CAD build for the part. Positions are in the model's coordinates, mm. Give positions to 0.01 mm unless a question says otherwise; leave off trailing zeros. Order: outer loops, then holes, each group sorted by start corner. A loop starts at its lowest first (then second) coordinate and runs counter-clockwise, first axis right, second up. Notation, with made-up numbers: (77.25, 62.25) -> (101.25, 62.25) arc R16 ccw to (101.25, 91.25) -> close; hole circle Ø10 at (58.5, -7). An arc over 180 degrees is marked (long way). Use one line per item in the form item = value. Start each with the question number.
1) Probe line 1 (Z direction, x = -0.6, y = -38.5). List the from-to ranges inside material, lowest first.
2) Cut at B-B, the plane x = -0.45. Give the cut face in (y, z), and give its area (3 significant figures).
3) Cut at A-A, the plane y = -64.5. Give the cut face in (x, z).
4) Cut at C-C, the plane z = -132. Give the cut face in (x, y).
Autodesk Inventor part; units mm, degrees
ref_plane "YZ Plane" through (0, 0, 0) normal (1, 0, 0) x (0, 1, 0)
ref_plane "XZ Plane" through (0, 0, 0) normal (0, 1, 0) x (-1, 0, 0)
ref_plane "XY Plane" through (0, 0, 0) normal (0, 0, 1) x (1, 0, 0)
sketch "Boceto1" plane through (0, 0, 0) normal (1, 0, 0) x (0, 1, 0)
  line L0 (13.0609, 21.0882) -> (-181.9391, 21.0882)
  line L1 (-181.9391, -279.9118) -> (13.0609, -279.9118)
  line L2 (13.0609, -279.9118) -> (13.0609, 21.0882)
  line L3 (-1.9391, -129.4118) -> (-1.9391, -154.4118)
  line L4 (-1.9391, -154.4118) -> (-181.9391, -154.4118)
  line L5 (-1.9391, -129.4118) -> (-1.9391, -104.4118)
  line L6 (-1.9391, -104.4118) -> (-181.9391, -104.4118)
  line L7 (-181.9391, 21.0882) -> (-181.9391, -104.4118)
  line L8 (-181.9391, -154.4118) -> (-181.9391, -279.9118)
  point P0 (0, 0)
  dimension "d0" = 195
  dimension "d1" = 301
  dimension "d3" = 25
  dimension "d4" = 25
extrude "Extrusión1" add sketch "Boceto1" along normal mid plane 1.5
properties part number "panel frontal"
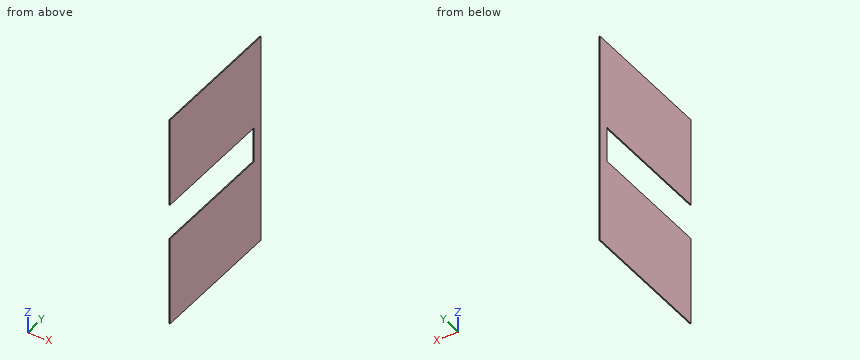
Result:
q1.line_1 = -279.91 to -154.41, -104.41 to 21.09
q2.outline = (-181.94, -279.91) -> (13.06, -279.91) -> (13.06, 21.09) -> (-181.94, 21.09) -> (-181.94, -104.41) -> (-1.94, -104.41) -> (-1.94, -154.41) -> (-181.94, -154.41) -> close
q2.area = 49,700 mm²
q3.outline = (-0.75, -279.91) -> (0.75, -279.91) -> (0.75, -154.41) -> (-0.75, -154.41) -> close; (-0.75, -104.41) -> (0.75, -104.41) -> (0.75, 21.09) -> (-0.75, 21.09) -> close
q4.outline = (-0.75, -1.94) -> (0.75, -1.94) -> (0.75, 13.06) -> (-0.75, 13.06) -> close
